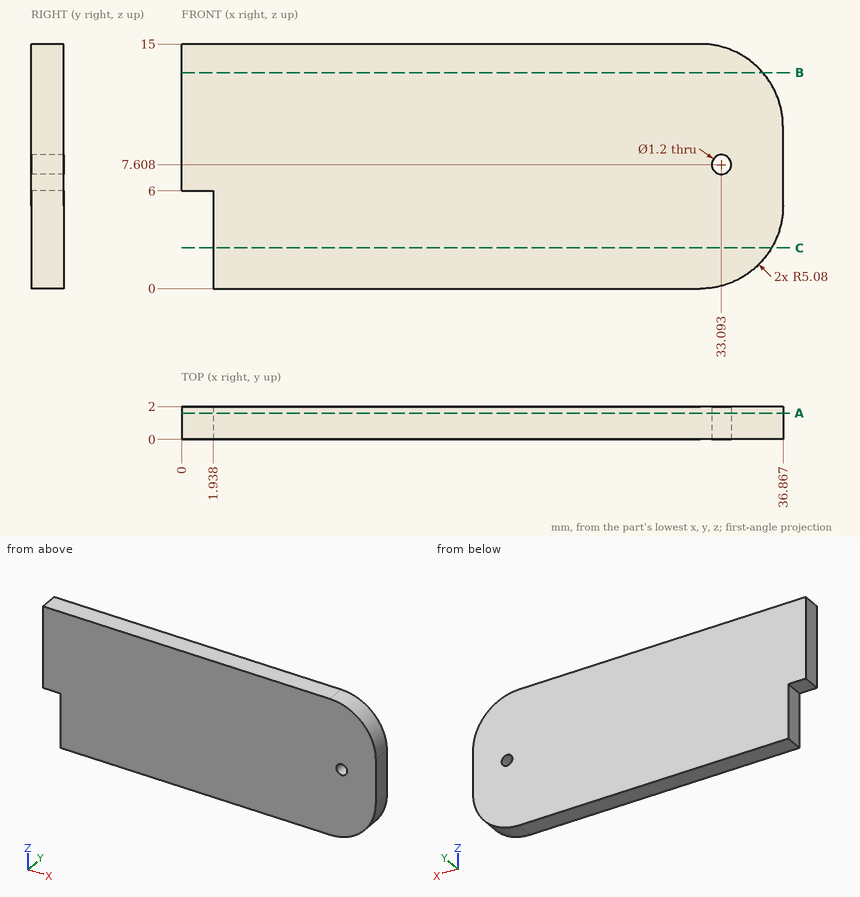
The drawing under review shows one solid part. Ordinate dimensions are in mm from its lowest x, y, z. Coordinates: 2 decimals unless noted, no trailing zeros. Loops run counter-clockwise (first coordinate to the right, second up) from the corner with the lowest first, then second, coordinate; pieces in that order, holes last.
Item 1: Add section B-B (z = 13.25). Write out the cut boundary in (x, y).
Completed:
outline: (0, 0) - (35.62, 0) - (35.62, 2) - (0, 2) - close
Item 2: Wall thickness on L1, parallel to X at y = 1, z = 5.75; L2, parallel to X at y = 1.7, z = 10.5: over which ranges is each line inside the solid? List them lowest first.
Completed:
L1: x = 1.94 to 36.87
L2: x = 0 to 36.83
Item 3: Add section C-C (z = 2.5). Write out the cut boundary in (x, y).
Completed:
outline: (1.94, 0) - (36.16, 0) - (36.16, 2) - (1.94, 2) - close
Item 4: Add section A-A (y = 1.6). Write out the cut boundary in (x, z), and give its area (3 significant figures).
Completed:
outline: (0, 6) - (1.94, 6) - (1.94, 0) - (31.79, 0) arc R5.08 ccw to (36.87, 5.08) - (36.87, 9.92) arc R5.08 ccw to (31.79, 15) - (0, 15) - close; hole circle Ø1.2 at (33.09, 7.61)
area: 529 mm2
Item 5: Clearance check with a flat-ended pin moving along its axis: pin 1 (1 mm diameter, centred on x = 1, y = 1.5, fed in from -Z). State where the tip first meets the part, or that it passes through.
Completed:
pin 1: stops at z = 6
